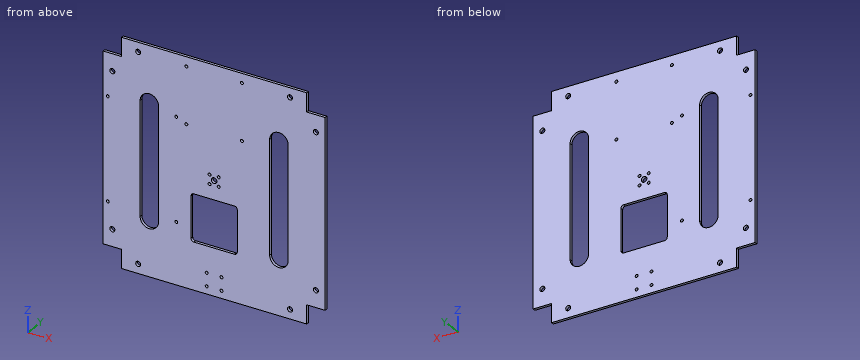
```python
from build123d import *

# Parameters (mm, degrees)
SKETCH_1_W          = 239.8
SKETCH_1_H          = 239.8
SKETCH_1_R          = 3
SKETCH_1_R_2        = 1.6
EXTRUDE_1_DEPTH     = 3
SKETCH_2_R          = 1.6
SKETCH_2_W          = 19.9
SKETCH_2_H          = 19.9
CUT_EXTRUDE_2_DEPTH = 3
SKETCH_3_R          = 1.6
CUT_EXTRUDE_3_DEPTH = 3
SKETCH_4_W          = 50
SKETCH_4_H          = 50
CUT_EXTRUDE_4_DEPTH = 3
FILLET_1_R          = 3
SKETCH_5_R          = 2.7
CUT_EXTRUDE_5_DEPTH = 3
SKETCH_6_R          = 1.6
CUT_EXTRUDE_7_DEPTH = 3


with BuildPart() as part:
    # 草图1 → 凸台-拉伸1 (new body)
    with BuildSketch(Plane(origin=(0, 0, 0), x_dir=(1, 0, 0), z_dir=(0, 1, 0))):
        Rectangle(SKETCH_1_W, SKETCH_1_H)
        with Locations(Location((0, 0, 0), (0, 0, 270))):
            Circle(SKETCH_1_R, mode=Mode.SUBTRACT)
        with Locations(Location((4.949747468, 4.949747468, 0), (0, 0, 270))):
            Circle(SKETCH_1_R_2, mode=Mode.SUBTRACT)
        with Locations(Location((4.949747468, -4.949747468, 0), (0, 0, 270))):
            Circle(SKETCH_1_R_2, mode=Mode.SUBTRACT)
        with Locations(Location((-4.949747468, -4.949747468, 0), (0, 0, 270))):
            Circle(SKETCH_1_R_2, mode=Mode.SUBTRACT)
        with Locations(Location((-4.949747468, 4.949747468, 0), (0, 0, 270))):
            Circle(SKETCH_1_R_2, mode=Mode.SUBTRACT)
    extrude(amount=EXTRUDE_1_DEPTH)

    # 草图2 → 切除-拉伸2 (cut)
    with BuildSketch(Plane(origin=(0, 3, 0), x_dir=(1, 0, 0), z_dir=(0, 1, 0))):
        with Locations(Location((-8, 111.9, 0), (0, 0, 270))):
            Circle(SKETCH_2_R)
        with Locations(Location((8, 111.9, 0), (0, 0, 90))):
            Circle(SKETCH_2_R)
        with Locations(Location((8, 97.9, 0), (0, 0, 270))):
            Circle(SKETCH_2_R)
        with Locations(Location((-8, 97.9, 0), (0, 0, 90))):
            Circle(SKETCH_2_R)
        with Locations((109.95, 109.95)):
            Rectangle(SKETCH_2_W, SKETCH_2_H)
        with Locations((-109.95, 109.95)):
            Rectangle(SKETCH_2_W, SKETCH_2_H)
        with Locations((109.95, -109.95)):
            Rectangle(SKETCH_2_W, SKETCH_2_H)
        with Locations((-109.95, -109.95)):
            Rectangle(SKETCH_2_W, SKETCH_2_H)
    extrude(amount=-CUT_EXTRUDE_2_DEPTH, mode=Mode.SUBTRACT)

    # 草图3 → 切除-拉伸3 (cut)
    with BuildSketch(Plane(origin=(0, 3, 0), x_dir=(1, 0, 0), z_dir=(0, 1, 0))):
        with Locations(Location((-30, -49.9, 0), (0, 0, 270))):
            Circle(SKETCH_3_R)
        with Locations(Location((30, -49.9, 0), (0, 0, 90))):
            Circle(SKETCH_3_R)
        with Locations(Location((-30, -109.9, 0), (0, 0, 90))):
            Circle(SKETCH_3_R)
        with Locations(Location((30, -109.9, 0), (0, 0, 270))):
            Circle(SKETCH_3_R)
    extrude(amount=-CUT_EXTRUDE_3_DEPTH, mode=Mode.SUBTRACT)

    # 草图4 → 切除-拉伸4 (cut)
    with BuildSketch(Plane(origin=(0, 3, 0), x_dir=(1, 0, 0), z_dir=(0, 1, 0))):
        with BuildLine():
            Line((-60, 60), (-60, -60))
            ThreePointArc((-60, -60), (-70, -70), (-80, -60))
            Line((-80, -60), (-80, 60))
            ThreePointArc((-80, 60), (-70, 70), (-60, 60))
        make_face()
        with BuildLine():
            Line((80, 60), (80, -60))
            ThreePointArc((80, -60), (70, -70), (60, -60))
            Line((60, -60), (60, 60))
            ThreePointArc((60, 60), (70, 70), (80, 60))
        make_face()
        with Locations((0, 45)):
            Rectangle(SKETCH_4_W, SKETCH_4_H)
    extrude(amount=-CUT_EXTRUDE_4_DEPTH, mode=Mode.SUBTRACT)

    # 圆角1
    fillet_1_edges = [part.edges().sort_by_distance(p)[0] for p in [
        (25, 1.5, -70),
        (25, 1.5, -20),
        (-25, 1.5, -20),
        (-25, 1.5, -70),
    ]]
    fillet(fillet_1_edges, radius=FILLET_1_R)

    # 草图5 → 切除-拉伸5 (cut)
    with BuildSketch(Plane(origin=(0, 3, 0), x_dir=(1, 0, 0), z_dir=(0, 1, 0))):
        with Locations(Location((-109.95, 82, 0), (0, 0, 270))):
            Circle(SKETCH_5_R)
        with Locations(Location((-82, 109.95, 0), (0, 0, 90))):
            Circle(SKETCH_5_R)
        with Locations(Location((-109.95, -82, 0), (0, 0, 90))):
            Circle(SKETCH_5_R)
        with Locations(Location((-82, -109.95, 0), (0, 0, 270))):
            Circle(SKETCH_5_R)
        with Locations(Location((109.95, 82, 0), (0, 0, 90))):
            Circle(SKETCH_5_R)
        with Locations(Location((82, 109.95, 0), (0, 0, 270))):
            Circle(SKETCH_5_R)
        with Locations(Location((109.95, -82, 0), (0, 0, 270))):
            Circle(SKETCH_5_R)
        with Locations(Location((82, -109.95, 0), (0, 0, 90))):
            Circle(SKETCH_5_R)
    extrude(amount=-CUT_EXTRUDE_5_DEPTH, mode=Mode.SUBTRACT)

    # 草图6 → 切除-拉伸7 (cut)
    with BuildSketch(Plane(origin=(0, 3, 0), x_dir=(1, 0, 0), z_dir=(0, 1, 0))):
        with Locations(Location((-114.9, 54.5, 0), (0, 0, 270))):
            Circle(SKETCH_6_R)
        with Locations(Location((-40.9, 54.5, 0), (0, 0, 270))):
            Circle(SKETCH_6_R)
        with Locations(Location((-114.9, -54.5, 0), (0, 0, 90))):
            Circle(SKETCH_6_R)
        with Locations(Location((-40.9, -54.5, 0), (0, 0, 270))):
            Circle(SKETCH_6_R)
    extrude(amount=-CUT_EXTRUDE_7_DEPTH, mode=Mode.SUBTRACT)


solid = part.part
```
The model under review builds one solid part; all positions refer to its coordinate system, in mm. Round coordinates to 2 decimals unless told otherwise and drop trailing zeros. Order: outer loops, then holes, each group sorted by start corner. A loop starts at its lowest first (then second) coordinate and runs counter-clockwise, first axis right, second up.
Item 1: To check wall thickness, follow probe 1 along X at (y, z) = (1.85, -12); probe 2 along X at (y, z) = (0.65, -52); probe 3 along X at (y, z) = (1.05, -82). State the ranges of each line that lie inside material, in increasing order.
Working result:
probe 1: x = -119.9 to -80, -60 to 60, 80 to 119.9
probe 2: x = -119.9 to -80, -60 to -25, 25 to 60, 80 to 119.9
probe 3: x = -119.9 to -112.65, -107.25 to 107.25, 112.65 to 119.9
Item 2: Add section C-C, the plane y = 1.95. Count the separate pieces of the cut face and the enclosed holes in it, and give its area (3 significant figures).
Working result:
separate pieces: 1
enclosed holes: 28
area: 47,700 mm2
Item 3: Add section B-B, the plane z = -63. State the section outline as (x, y) points.
Working result:
outline: (-119.9, 0) - (-79.54, 0) - (-79.54, 3) - (-119.9, 3) - close; (-60.46, 0) - (-25, 0) - (-25, 3) - (-60.46, 3) - close; (25, 0) - (60.46, 0) - (60.46, 3) - (25, 3) - close; (79.54, 0) - (119.9, 0) - (119.9, 3) - (79.54, 3) - close
Item 4: Add section A-A, the plane z = -30. State the section outline as (x, y) points, and give its area (3 significant figures).
Working result:
outline: (-119.9, 0) - (-80, 0) - (-80, 3) - (-119.9, 3) - close; (-60, 0) - (-25, 0) - (-25, 3) - (-60, 3) - close; (25, 0) - (60, 0) - (60, 3) - (25, 3) - close; (80, 0) - (119.9, 0) - (119.9, 3) - (80, 3) - close
area: 449 mm2
